The figure shows three views and two pictorial views of one solid part (mm, origin at its lowest corner). Answer the questions. Coordinates: 2 decimals unless noted, no trailing zeros. Order: outer loops, then holes, each group sorted by start corner. A loop starts at its lowest first (then second) coordinate and runs counter-clockwise, first axis right, second up. Notation, with made-up numbers: (8, -37.75) -> (58, -37.75) arc R22 cw to (58, -22.75) -> close; hole circle Ø8 at (-7, -27). An arc over 180 degrees is marked (long way). Return JSON: item names as keys, results as strings.
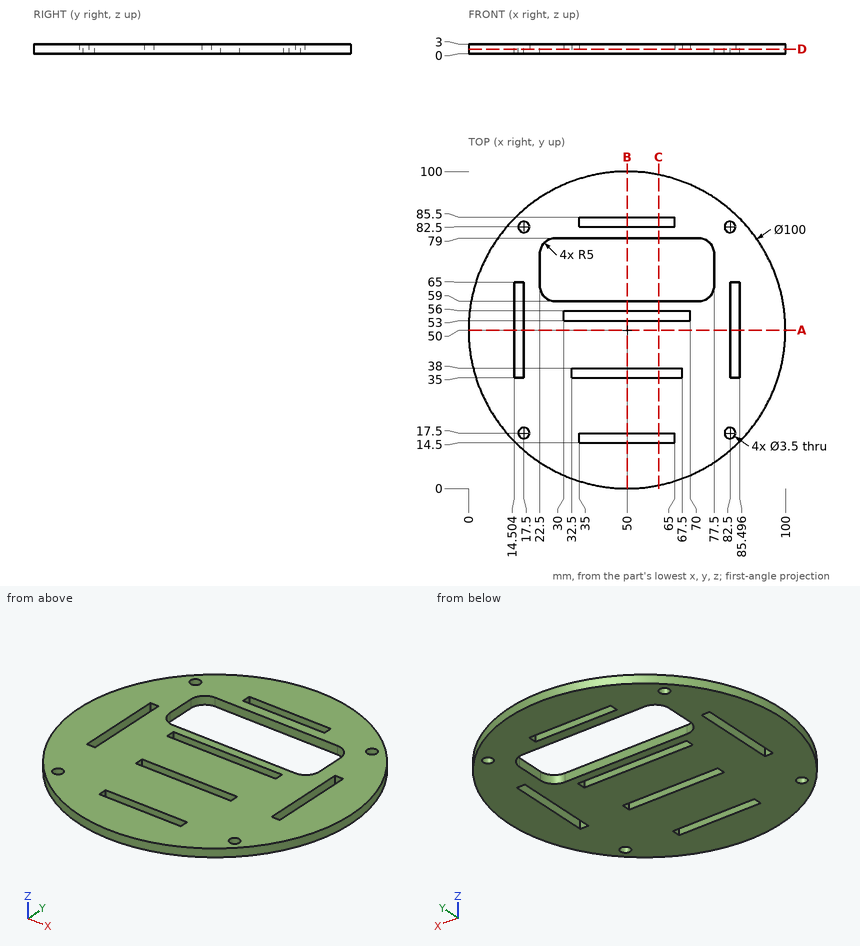
Item 1: Find the intervals of material crossed by probe 1 along Y at (x, z) = (64, 1.85); probe 2 along X at (y, z) = (81, 2); probe 3 along X at (y, z) = (18.5, 1.5) (1 decimal), in increasing order.
Answer list:
{"probe 1": "2 to 14.5, 17.5 to 35, 38 to 53, 56 to 59, 79 to 82.5, 85.5 to 98", "probe 2": "10.77 to 16.6, 18.4 to 81.6, 83.4 to 89.23", "probe 3": "11.2 to 16.1, 18.9 to 81.1, 83.9 to 88.8"}
Item 2: The part is cut by section A-A on y = 50. Determine the outline of the cut face in (x, z), plus the area to 3 significant figures.
Answer list:
{"outline": "(0, 0) -> (14.5, 0) -> (14.5, 3) -> (0, 3) -> close; (17.5, 0) -> (82.5, 0) -> (82.5, 3) -> (17.5, 3) -> close; (85.5, 0) -> (100, 0) -> (100, 3) -> (85.5, 3) -> close", "area": "282 mm2"}
Item 3: The part is cut by section B-B on x = 50. Determine the outline of the cut face in (y, z).
Answer list:
{"outline": "(0, 0) -> (14.5, 0) -> (14.5, 3) -> (0, 3) -> close; (17.5, 0) -> (35, 0) -> (35, 3) -> (17.5, 3) -> close; (38, 0) -> (53, 0) -> (53, 3) -> (38, 3) -> close; (56, 0) -> (59, 0) -> (59, 3) -> (56, 3) -> close; (79, 0) -> (82.5, 0) -> (82.5, 3) -> (79, 3) -> close; (85.5, 0) -> (100, 0) -> (100, 3) -> (85.5, 3) -> close"}
Item 4: Flat-ended cylindrical pins translate along their axes: pin 1 (0.9 mm diameter, centred on y = 46, z = 2, fed in from +X); pin 2 (1.5 mm diameter, centred on x = 83.5, z = 2, fed in from +Y); pin 3 (0.9 mm diameter, centred on x = 15.5, z = 1, fed in from +Y) (1 decimal); pin 4 (10 mm diameter, centred on x = 84.5, y = 14, fed in from -Z). Find the tip coordinate at first contact, or state that the pin passes through.
Answer list:
{"pin 1": "x = 99.87", "pin 2": "y = 87.78", "pin 3": "y = 86.6", "pin 4": "z = 0"}
Item 5: The part is cut by section C-C on x = 60. Determine the outline of the cut face in (y, z), plus the area to 3 significant figures.
Answer list:
{"outline": "(1.01, 0) -> (14.5, 0) -> (14.5, 3) -> (1.01, 3) -> close; (17.5, 0) -> (35, 0) -> (35, 3) -> (17.5, 3) -> close; (38, 0) -> (53, 0) -> (53, 3) -> (38, 3) -> close; (56, 0) -> (59, 0) -> (59, 3) -> (56, 3) -> close; (79, 0) -> (82.5, 0) -> (82.5, 3) -> (79, 3) -> close; (85.5, 0) -> (98.99, 0) -> (98.99, 3) -> (85.5, 3) -> close", "area": "198 mm2"}
Item 6: The part is cut by section D-D on z = 1.4. Count the separate pieces of the cut face and the enclosed holes in it, plus the area to 3 significant figures.
Answer list:
{"separate pieces": "1", "enclosed holes": "11", "area": "6,150 mm2"}
